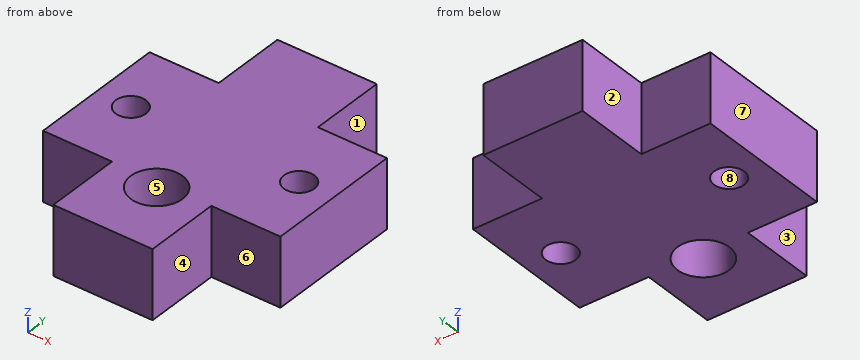
from build123d import *

# Parameters (mm, degrees)
SKETCH1_W           = 6.4
SKETCH1_H           = 12.7
SKETCH1_R           = 1.4
BOSS_EXTRUDE1_DEPTH = 6.35
SKETCH2_R           = 2.4
CUT_EXTRUDE1_DEPTH  = 19.426746864


with BuildPart() as part:
    # Sketch1 → Boss-Extrude1 (new body)
    # profile 1 of 5: a face of its own
    with BuildSketch(Plane.XY):
        Polygon((-4.6, 13.35), (-4.6, 6.35), (-4.6, -6.35), (-4.6, -13.35), (4.6, -13.35), (4.6, -6.35), (4.6, 6.35), (4.6, 13.35), align=None)
    # profile 2 of 5: a face of its own
    with BuildSketch(Plane.XY):
        Polygon((-4.6, 13.35), (-4.6, 6.35), (-4.6, -6.35), (-4.6, -13.35), (4.6, -13.35), (4.6, -6.35), (4.6, 6.35), (4.6, 13.35), align=None)
    # profile 3 of 5: a face of its own
    with BuildSketch(Plane.XY):
        Polygon((-4.6, 13.35), (-4.6, 6.35), (-4.6, -6.35), (-4.6, -13.35), (4.6, -13.35), (4.6, -6.35), (4.6, 6.35), (4.6, 13.35), align=None)
    # profile 4 of 5: a face of its own
    with BuildSketch(Plane.XY):
        with Locations((7.8, 0)):
            Rectangle(SKETCH1_W, SKETCH1_H)
        with Locations((7.8, 0)):
            Circle(SKETCH1_R, mode=Mode.SUBTRACT)
    # profile 5 of 5: a face of its own
    with BuildSketch(Plane.XY):
        with Locations((-7.8, 0)):
            Rectangle(SKETCH1_W, SKETCH1_H)
        with Locations((-7.8, 0)):
            Circle(SKETCH1_R, mode=Mode.SUBTRACT)
    extrude(amount=BOSS_EXTRUDE1_DEPTH)

    # Sketch2 → Cut-Extrude1 (cut, through all)
    with BuildSketch(Plane(origin=(0, 0, 0), x_dir=(-1, 0, 0), z_dir=(0, 0, -1))):
        with Locations((0, -6.95)):
            Circle(SKETCH2_R)
    extrude(amount=-CUT_EXTRUDE1_DEPTH, mode=Mode.SUBTRACT)


solid = part.part
Part model, mm, in its own coordinate system. Face numbers are marked on the shaded views. A direction names the side the tool comes from. Coordinates: 2 decimals unless noted, no trailing zeros. Loops run counter-clockwise (first coordinate to the right, second up) from the corner with the lowest first, then second, coordinate; pieces in that order, holes last. Notation, with made-up numbers: (-6, 21) -> (5, 21) arc R14 ccw to (5, 39) -> close; hole circle Ø11 at (12, -5.5). An arc over 180 degrees is marked (long way). Use a Markdown table: item, result. Add a question column.
Item 1: Flat gauge pins, fed straight in: P1, Ø1.9, axis at y = 11.5, z = 3, coming from the +X side; P2, Ø1.7, axis at x = -7.8, y = 0, coming from the +Z side; P3, Ø3, axis at y = -10.5, z = 3, coming from the -X side. Where does each tip first touch, or does it go through?
Item 2: Band-saw the part on A-A on x = 7.8. Write the cut outline in (y, z), plus the area to 3 significant figures.
Item 3: Probe probe 1 along Y at (x, z) = (-7.8, 4); probe 2 along Y at (x, z) = (0, 3); probe 3 along Y at (x, z) = (6, 6). List the from-to ranges inside material, lowest first.
Item 4: Band-saw the part on D-D on z = 2. Write the cut outline in (x, y).
Item 5: Pull direction X, two halves, no side cores. Call the marked faces 6, 7 and 8: +X half, -X half, draft (parallel to the pull), parting line (faces both ways), or undercut.
Item 6: Band-saw the part on C-C on y = -6.95. Write the cut outline in (x, z).
Item 7: Which spindle directions (+Z, -Z, +X, -X, +Y, -Y) get a long thin tool onto all of the face, cutting with end or side? Do the marked faces 1, 2, 3, 4 and 5. Say none if no direction does.
Item 8: Band-saw the part on B-B on y = 0. Write the cut outline in (x, z), plus the area to 3 significant figures.
Geometry says:
| question | item | result |
|---|---|---|
| 1 | P1 | x = 4.6 |
| 1 | P2 | through |
| 1 | P3 | x = -4.6 |
| 2 | outline | (-6.35, 0) -> (-1.4, 0) -> (-1.4, 6.35) -> (-6.35, 6.35) -> close; (1.4, 0) -> (6.35, 0) -> (6.35, 6.35) -> (1.4, 6.35) -> close |
| 2 | area | 62.9 mm² |
| 3 | probe 1 | -6.35 to -1.4, 1.4 to 6.35 |
| 3 | probe 2 | -13.35 to -9.35, -4.55 to 13.35 |
| 3 | probe 3 | -6.35 to 6.35 |
| 4 | outline | (-11, -6.35) -> (-4.6, -6.35) -> (-4.6, -13.35) -> (4.6, -13.35) -> (4.6, -6.35) -> (11, -6.35) -> (11, 6.35) -> (4.6, 6.35) -> (4.6, 13.35) -> (-4.6, 13.35) -> (-4.6, 6.35) -> (-11, 6.35) -> close; hole circle Ø2.8 at (-7.8, 0); hole circle Ø4.8 at (0, -6.95); hole circle Ø2.8 at (7.8, 0) |
| 5 | face 6 | draft |
| 5 | face 7 | -X half |
| 5 | face 8 | undercut |
| 6 | outline | (-4.6, 0) -> (-2.4, 0) -> (-2.4, 6.35) -> (-4.6, 6.35) -> close; (2.4, 0) -> (4.6, 0) -> (4.6, 6.35) -> (2.4, 6.35) -> close |
| 7 | face 1 | +Z, -Z, +X, +Y |
| 7 | face 2 | +Z, -Z, -X, +Y |
| 7 | face 3 | +Z, -Z, -X, -Y |
| 7 | face 4 | +Z, -Z, +X, -Y |
| 7 | face 5 | +Z, -Z |
| 8 | outline | (-11, 0) -> (-9.2, 0) -> (-9.2, 6.35) -> (-11, 6.35) -> close; (-6.4, 0) -> (6.4, 0) -> (6.4, 6.35) -> (-6.4, 6.35) -> close; (9.2, 0) -> (11, 0) -> (11, 6.35) -> (9.2, 6.35) -> close |
| 8 | area | 104 mm² |
